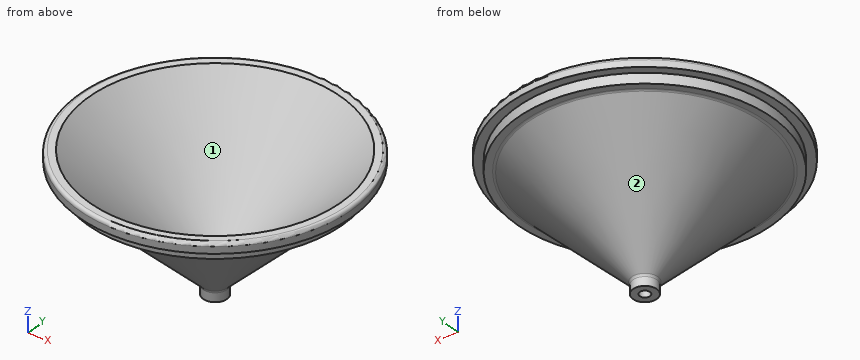
```python
from build123d import *

# Parameters (mm, degrees)
FILLET009_R = 1
FILLET010_R = 1
FILLET011_R = 1
FILLET012_R = 1


with BuildPart() as part:
    # Sketch044 → Revolution (revolve)
    with BuildSketch(Plane.XZ):
        Polygon((40, 61), (40, 58), (37.5, 58), (37.5, 55), (35, 55), (3.5, 24), (3.5, 21), (1.5, 21), (1.5, 25.5), (37, 61), align=None)
    revolve(axis=Axis((0, 0, 0), (0, 0, 1)))

    # Fillet009
    fillet009_edges = [part.edges().sort_by_distance(p)[0] for p in [
        (-1.5, 0, 25.5),
    ]]
    fillet(fillet009_edges, radius=FILLET009_R)

    # Fillet010
    fillet010_edges = [part.edges().sort_by_distance(p)[0] for p in [
        (-40, 0, 61),
    ]]
    fillet(fillet010_edges, radius=FILLET010_R)

    # Fillet011
    fillet011_edges = [part.edges().sort_by_distance(p)[0] for p in [
        (-3.5, 0, 24),
    ]]
    fillet(fillet011_edges, radius=FILLET011_R)

    # Fillet012
    fillet012_edges = [part.edges().sort_by_distance(p)[0] for p in [
        (-35, 0, 55),
    ]]
    fillet(fillet012_edges, radius=FILLET012_R)


with BuildPart() as part_1:
    # Body006 placement: moved
    add(part.part.moved(Location((0, 0, 1))))


solid = part_1.part
```
Model file for the job. Use its own axes, mm. Face numbers are marked on the shaded views. Coordinates: 2 decimals unless noted, no trailing zeros. Loops run counter-clockwise (first coordinate to the right, second up) from the corner with the lowest first, then second, coordinate; pieces in that order, holes last. Notation, with made-up numbers: (51.5, 72.5) -> (86.5, 72.5) arc R29 ccw to (86.5, 108.5) -> close; hole circle Ø10 at (42.25, -3). An arc over 180 degrees is marked (long way). Answer as a JSON object with one key per item and string values.
Q1. Pull direction Y, two halves, no side cores. Call the marked faces 1 and 2: released by +Y, released by -Y, zero draft, split by the parting line, or undercut.
Report:
{"face 1": "undercut", "face 2": "split by the parting line"}
Q2. Cut at A-A (z = 29). List the corners of the cut face in (x, y), and give its area (3 significant figures).
Report:
{"outline": "circle Ø15.13 at (0, 0); hole circle Ø8 at (0, 0)", "area": "130 mm2"}
Q3. Flat gauge pins, fed straight in: P1, Ø4, axis at x = 31, y = 13, coming from the +Z side; P2, Ø1.5, axis at y = -0.5, z = 36, coming from the +X side; P3, Ø1.5, axis at y = 19.5, z = 56.5, coming from the -X side. Where does each tip first touch, or does it go through?
Report:
{"P1": "stops at z = 60.62", "P2": "stops at x = 15.43", "P3": "stops at x = -32.48"}
Q4. Probe probe 1 along X at (y, z) = (0, 24.4); probe 2 along Y at (x, z) = (-8, 45.5). List the from-to ranges inside material, lowest first.
Report:
{"probe 1": "x = -3.5 to -1.5, 1.5 to 3.5", "probe 2": "y = -22.98 to -18.87, 18.87 to 22.98"}
Q5. Cut at B-B (z = 38). List the corners of the cut face in (x, y).
Report:
{"outline": "circle Ø33.42 at (0, 0); hole circle Ø26 at (0, 0)"}
